For this review, take the finished solid that the model builds, in its own axes (mm). A direction names the side the tool comes from. Round coordinates to 2 decimals unless told otherwise and drop trailing zeros. Order: outer loops, then holes, each group sorted by start corner. A loop starts at its lowest first (then second) coordinate and runs counter-clockwise, first axis right, second up. Notation, with made-up numbers: M 73.5,-22.5 L 98.5,-22.5 A28 cw 98.5,14.5 Z; hole C -4.5,-20.5 d4. An arc over 180 degrees is marked long. Put each result on its own line as item: value.
from build123d import *

# Parameters (mm, degrees)
BOSS_EXTRUDE1_DEPTH = 9.95
SKETCH2_W           = 58
SKETCH2_H           = 9.95
BOSS_EXTRUDE2_DEPTH = 8.55
SKETCH3_W           = 9.8
SKETCH3_H           = 11.55
BOSS_EXTRUDE3_DEPTH = 4
BOSS_EXTRUDE4_DEPTH = 20
CHAMFER1_SIZE       = 2
CUT_EXTRUDE1_REACH  = 70.57
CHAMFER2_SIZE       = 1
BOSS_EXTRUDE5_DEPTH = 5
CHAMFER3_SIZE       = 2
SKETCH7_W           = 10
SKETCH7_H           = 20
CUT_EXTRUDE2_DEPTH  = 7
CHAMFER4_SIZE       = 2
CHAMFER5_SIZE       = 1
SKETCH8_R           = 1.25
CUT_EXTRUDE3_DEPTH  = 15
CHAMFER6_SIZE       = 1.5
CHAMFER7_SIZE       = 2


with BuildPart() as part:
    # Sketch1 → Boss-Extrude1 (new body)
    with BuildSketch(Plane(origin=(0, 0, 0), x_dir=(1, 0, 0), z_dir=(0, 1, 0))):
        with BuildLine():
            Line((-10.05, -13), (-19.52904451, -13))
            ThreePointArc((-19.52904451, -13), (-23.22122875, -23.900809511), (-29, -33.853983643))
            Line((-29, -33.853983643), (-29, -45))
            Line((-29, -45), (29, -45))
            Line((29, -45), (29, -33.853983643))
            ThreePointArc((29, -33.853983643), (23.22122875, -23.900809511), (19.52904451, -13))
            Line((19.52904451, -13), (10.05, -13))
            Line((10.05, -13), (10.05, -15.9))
            Line((10.05, -15.9), (18.25, -15.9))
            Line((18.25, -15.9), (18.25, -19.68))
            Line((18.25, -19.68), (10.05, -19.68))
            Line((10.05, -19.68), (10.05, -22.68))
            Line((10.05, -22.68), (18.360244512, -22.68))
            ThreePointArc((18.360244512, -22.68), (21.116099011, -28.699201931), (24.5, -34.389082421))
            Line((24.5, -34.389082421), (24.5, -42))
            Line((24.5, -42), (-24.5, -42))
            Line((-24.5, -42), (-24.5, -34.389082421))
            ThreePointArc((-24.5, -34.389082421), (-21.116099011, -28.699201931), (-18.360244512, -22.68))
            Line((-18.360244512, -22.68), (-10.05, -22.68))
            Line((-10.05, -22.68), (-10.05, -19.68))
            Line((-10.05, -19.68), (-18.25, -19.68))
            Line((-18.25, -19.68), (-18.25, -15.9))
            Line((-18.25, -15.9), (-10.05, -15.9))
            Line((-10.05, -15.9), (-10.05, -13))
        make_face()
    extrude(amount=BOSS_EXTRUDE1_DEPTH)

    # Sketch2 → Boss-Extrude2 (add)
    with BuildSketch(Plane.XY.offset(45)):
        with Locations((0, 4.975)):
            Rectangle(SKETCH2_W, SKETCH2_H)
    extrude(amount=BOSS_EXTRUDE2_DEPTH)

    # Sketch3 → Boss-Extrude3 (add)
    with BuildSketch(Plane(origin=(0, 9.95, 0), x_dir=(1, 0, 0), z_dir=(0, 1, 0))):
        with Locations((0, -47.775)):
            Rectangle(SKETCH3_W, SKETCH3_H)
    extrude(amount=BOSS_EXTRUDE3_DEPTH)

    # Sketch4 → Boss-Extrude4 (add)
    with BuildSketch(Plane.XY.offset(53.55)):
        Polygon((-29, 9.95), (-29, 0), (29, 0), (29, 9.95), (4.9, 9.95), (4.9, 13.95), (-4.9, 13.95), (-4.9, 9.95), align=None)
    extrude(amount=BOSS_EXTRUDE4_DEPTH)

    # Chamfer1
    chamfer1_edges = [part.edges().sort_by_distance(p)[0] for p in [
        (4.9, 11.95, 42),
        (-4.9, 11.95, 42),
    ]]
    chamfer(chamfer1_edges, length=CHAMFER1_SIZE)

    # Cut-Extrude1: up to this face of the body (flat: up to its plane)
    cut_extrude1_end = Plane(part.part.faces().sort_by_distance((14.205122256, 4.975, 22.68))[0])
    # Sketch5 → Cut-Extrude1 (cut, up to the picked face)
    with BuildSketch(Plane(origin=(0, 0, 13), x_dir=(-1, 0, 0), z_dir=(0, 0, -1)), mode=Mode.PRIVATE) as cut_extrude1_sk1:
        with BuildLine():
            ThreePointArc((-14.25, 4.975), (-13, 3.725), (-11.75, 4.975))
            Line((-11.75, 4.975), (-14.25, 4.975))
        make_face()
    cut_extrude1_tool1 = split(extrude(cut_extrude1_sk1.sketch, amount=-CUT_EXTRUDE1_REACH, mode=Mode.PRIVATE), bisect_by=cut_extrude1_end, keep=Keep.BOTH, mode=Mode.PRIVATE)
    # Sketch5 → Cut-Extrude1 (cut, up to the picked face)
    with BuildSketch(Plane(origin=(0, 0, 13), x_dir=(-1, 0, 0), z_dir=(0, 0, -1)), mode=Mode.PRIVATE) as cut_extrude1_sk2:
        with BuildLine():
            Line((-14.25, 4.975), (-11.75, 4.975))
            ThreePointArc((-11.75, 4.975), (-13, 6.225), (-14.25, 4.975))
        make_face()
    cut_extrude1_tool2 = split(extrude(cut_extrude1_sk2.sketch, amount=-CUT_EXTRUDE1_REACH, mode=Mode.PRIVATE), bisect_by=cut_extrude1_end, keep=Keep.BOTH, mode=Mode.PRIVATE)
    # Sketch5 → Cut-Extrude1 (cut, up to the picked face)
    with BuildSketch(Plane(origin=(0, 0, 13), x_dir=(-1, 0, 0), z_dir=(0, 0, -1)), mode=Mode.PRIVATE) as cut_extrude1_sk3:
        with BuildLine():
            ThreePointArc((-14.25, 4.975), (-13, 3.725), (-11.75, 4.975))
            Line((-11.75, 4.975), (-14.25, 4.975))
        make_face()
    cut_extrude1_tool3 = split(extrude(cut_extrude1_sk3.sketch, amount=-CUT_EXTRUDE1_REACH, mode=Mode.PRIVATE), bisect_by=cut_extrude1_end, keep=Keep.BOTH, mode=Mode.PRIVATE)
    # Sketch5 → Cut-Extrude1 (cut, up to the picked face)
    with BuildSketch(Plane(origin=(0, 0, 13), x_dir=(-1, 0, 0), z_dir=(0, 0, -1)), mode=Mode.PRIVATE) as cut_extrude1_sk4:
        with BuildLine():
            Line((-14.25, 4.975), (-11.75, 4.975))
            ThreePointArc((-11.75, 4.975), (-13, 6.225), (-14.25, 4.975))
        make_face()
    cut_extrude1_tool4 = split(extrude(cut_extrude1_sk4.sketch, amount=-CUT_EXTRUDE1_REACH, mode=Mode.PRIVATE), bisect_by=cut_extrude1_end, keep=Keep.BOTH, mode=Mode.PRIVATE)
    # Sketch5 → Cut-Extrude1 (cut, up to the picked face)
    with BuildSketch(Plane(origin=(0, 0, 13), x_dir=(-1, 0, 0), z_dir=(0, 0, -1)), mode=Mode.PRIVATE) as cut_extrude1_sk5:
        with BuildLine():
            ThreePointArc((14.25, 4.975), (13, 6.225), (11.75, 4.975))
            Line((11.75, 4.975), (14.25, 4.975))
        make_face()
    cut_extrude1_tool5 = split(extrude(cut_extrude1_sk5.sketch, amount=-CUT_EXTRUDE1_REACH, mode=Mode.PRIVATE), bisect_by=cut_extrude1_end, keep=Keep.BOTH, mode=Mode.PRIVATE)
    # Sketch5 → Cut-Extrude1 (cut, up to the picked face)
    with BuildSketch(Plane(origin=(0, 0, 13), x_dir=(-1, 0, 0), z_dir=(0, 0, -1)), mode=Mode.PRIVATE) as cut_extrude1_sk6:
        with BuildLine():
            Line((14.25, 4.975), (11.75, 4.975))
            ThreePointArc((11.75, 4.975), (13, 3.725), (14.25, 4.975))
        make_face()
    cut_extrude1_tool6 = split(extrude(cut_extrude1_sk6.sketch, amount=-CUT_EXTRUDE1_REACH, mode=Mode.PRIVATE), bisect_by=cut_extrude1_end, keep=Keep.BOTH, mode=Mode.PRIVATE)
    # Sketch5 → Cut-Extrude1 (cut, up to the picked face)
    with BuildSketch(Plane(origin=(0, 0, 13), x_dir=(-1, 0, 0), z_dir=(0, 0, -1)), mode=Mode.PRIVATE) as cut_extrude1_sk7:
        with BuildLine():
            ThreePointArc((14.25, 4.975), (13, 6.225), (11.75, 4.975))
            Line((11.75, 4.975), (14.25, 4.975))
        make_face()
    cut_extrude1_tool7 = split(extrude(cut_extrude1_sk7.sketch, amount=-CUT_EXTRUDE1_REACH, mode=Mode.PRIVATE), bisect_by=cut_extrude1_end, keep=Keep.BOTH, mode=Mode.PRIVATE)
    # Sketch5 → Cut-Extrude1 (cut, up to the picked face)
    with BuildSketch(Plane(origin=(0, 0, 13), x_dir=(-1, 0, 0), z_dir=(0, 0, -1)), mode=Mode.PRIVATE) as cut_extrude1_sk8:
        with BuildLine():
            Line((14.25, 4.975), (11.75, 4.975))
            ThreePointArc((11.75, 4.975), (13, 3.725), (14.25, 4.975))
        make_face()
    cut_extrude1_tool8 = split(extrude(cut_extrude1_sk8.sketch, amount=-CUT_EXTRUDE1_REACH, mode=Mode.PRIVATE), bisect_by=cut_extrude1_end, keep=Keep.BOTH, mode=Mode.PRIVATE)
    add(cut_extrude1_tool1.solids().sort_by(Axis((13, 4.444484, 13), (0, 0, 1)))[0], mode=Mode.SUBTRACT)
    add(cut_extrude1_tool2.solids().sort_by(Axis((13, 5.505516, 13), (0, 0, 1)))[0], mode=Mode.SUBTRACT)
    add(cut_extrude1_tool3.solids().sort_by(Axis((13, 4.444484, 13), (0, 0, 1)))[0], mode=Mode.SUBTRACT)
    add(cut_extrude1_tool4.solids().sort_by(Axis((13, 5.505516, 13), (0, 0, 1)))[0], mode=Mode.SUBTRACT)
    add(cut_extrude1_tool5.solids().sort_by(Axis((-13, 5.505516, 13), (0, 0, 1)))[0], mode=Mode.SUBTRACT)
    add(cut_extrude1_tool6.solids().sort_by(Axis((-13, 4.444484, 13), (0, 0, 1)))[0], mode=Mode.SUBTRACT)
    add(cut_extrude1_tool7.solids().sort_by(Axis((-13, 5.505516, 13), (0, 0, 1)))[0], mode=Mode.SUBTRACT)
    add(cut_extrude1_tool8.solids().sort_by(Axis((-13, 4.444484, 13), (0, 0, 1)))[0], mode=Mode.SUBTRACT)

    # Chamfer2
    chamfer2_edges = [part.edges().sort_by_distance(p)[0] for p in [
        (11.75, 4.975, 13),
        (-11.75, 4.975, 13),
    ]]
    chamfer(chamfer2_edges, length=CHAMFER2_SIZE)

    # Sketch6 → Boss-Extrude5 (add)
    with BuildSketch(Plane.XY.offset(73.55)):
        Polygon((29, 9.95), (29, 0), (38, 0), (38, 13.95), (4.9, 13.95), (4.9, 9.95), align=None)
        Polygon((-38, 13.95), (-38, 0), (-29, 0), (-29, 9.95), (-4.9, 9.95), (-4.9, 13.95), align=None)
    extrude(amount=-BOSS_EXTRUDE5_DEPTH)

    # Chamfer3
    chamfer3_edges = [part.edges().sort_by_distance(p)[0] for p in [
        (0, 13.95, 42),
        (3.9, 13.95, 43),
        (-3.9, 13.95, 43),
        (4.9, 13.95, 56.275),
        (33.5, 0, 68.55),
        (38, 0, 71.05),
        (38, 6.975, 68.55),
        (38, 13.95, 71.05),
        (4.9, 11.95, 68.55),
        (21.45, 13.95, 68.55),
        (-4.9, 13.95, 56.275),
        (-38, 13.95, 71.05),
        (-33.5, 0, 68.55),
        (-38, 0, 71.05),
        (-21.45, 13.95, 68.55),
        (-4.9, 11.95, 68.55),
        (-38, 6.975, 68.55),
    ]]
    chamfer(chamfer3_edges, length=CHAMFER3_SIZE)

    # Sketch7 → Cut-Extrude2 (cut)
    with BuildSketch(Plane(origin=(0, 9.95, 0), x_dir=(1, 0, 0), z_dir=(0, 1, 0))):
        with Locations((-14.9, -52)):
            Rectangle(SKETCH7_W, SKETCH7_H)
        with Locations((14.9, -52)):
            Rectangle(SKETCH7_W, SKETCH7_H)
    extrude(amount=-CUT_EXTRUDE2_DEPTH, mode=Mode.SUBTRACT)

    # Chamfer4
    chamfer4_edges = [part.edges().sort_by_distance(p)[0] for p in [
        (-9.9, 9.95, 52),
        (-9.9, 6.45, 42),
        (-9.9, 6.45, 62),
        (-19.9, 6.45, 62),
        (-19.9, 6.45, 42),
        (-19.9, 9.95, 52),
        (-14.9, 9.95, 62),
        (19.9, 9.95, 52),
        (19.9, 6.45, 42),
        (19.9, 6.45, 62),
        (9.9, 6.45, 62),
        (9.9, 6.45, 42),
        (9.9, 9.95, 52),
        (14.9, 9.95, 62),
    ]]
    chamfer(chamfer4_edges, length=CHAMFER4_SIZE)

    # Chamfer5
    chamfer5_edges = [part.edges().sort_by_distance(p)[0] for p in [
        (-24.5, 4.975, 42),
        (24.5, 4.975, 42),
    ]]
    chamfer(chamfer5_edges, length=CHAMFER5_SIZE)

    # Sketch8 → Cut-Extrude3 (cut)
    with BuildSketch(Plane.XY.offset(73.55)):
        with Locations((-25, 6.975)):
            Circle(SKETCH8_R)
        with Locations((25, 6.975)):
            Circle(SKETCH8_R)
        with Locations((0, 6.975)):
            Circle(SKETCH8_R)
    extrude(amount=-CUT_EXTRUDE3_DEPTH, mode=Mode.SUBTRACT)

    # Chamfer6
    chamfer6_edges = [part.edges().sort_by_distance(p)[0] for p in [
        (-29, 9.95, 51.201991821),
        (-14.789522255, 9.95, 13),
        (-23.22122875, 9.95, 23.900809511),
        (29, 9.95, 51.201991821),
        (23.22122875, 9.95, 23.900809511),
        (14.789522255, 9.95, 13),
    ]]
    chamfer(chamfer6_edges, length=CHAMFER6_SIZE)

    # Chamfer7
    chamfer7_edges = [part.edges().sort_by_distance(p)[0] for p in [
        (-14.9, 2.95, 42),
        (14.9, 2.95, 42),
    ]]
    chamfer(chamfer7_edges, length=CHAMFER7_SIZE)


solid = part.part
(1) Add section A-A on x = 13. State how many separate pieces and enclosed holes the cut face has, then the cut area to 3 significant figures.
A:
separate pieces: 5
enclosed holes: 0
area: 230 mm2
(2) For faces 4 (the face through (-12.08, 5.82, 14.94)), 5 (the face through (-32.55, 1.01, 69.54)), 6 (the face through (-15, 5, 62)), 7 (the face through (-28.26, 9.19, 51.44)), 8 (the face through (18.25, 5, 18)), list the 3-axis set-ups (+Z, -Z, +X, -X, +Y, -Y) from which the entire face can be reached by the end or side of a thin tool; tool diameter is ignored.
A:
face 4: -Z
face 5: -Z, -X, -Y
face 6: +Y
face 7: -Z, -X, +Y
face 8: +Y, -Y
(3) To check wall thickness, follow L1, parallel to Z at x = -16, y = 6.5; L2, parallel to X at y = 5, z = 49; L3, parallel to Y at x = -25, z = 68 (3 decimals). State the ranges of each line that lie inside material, in increasing order.
A:
L1: z = 13 to 15.9, 19.68 to 22.68, 62 to 73.55
L2: x = -29 to -19.9, -9.9 to 9.9, 19.9 to 29
L3: y = 0 to 5.725, 8.225 to 9.95
(4) Add section D-D on y = 13. Give the boundary of the cut face in (x, z).
A:
outline: M -36.95,70.55 L -36,69.6 L -6.9,69.6 L -3.85,66.55 L -3.85,44.43 L -2.47,43.05 L 2.47,43.05 L 3.85,44.43 L 3.85,66.55 L 6.9,69.6 L 36,69.6 L 36.95,70.55 L 36.95,73.55 L -36.95,73.55 Z
(5) Insertion check: pin 1 Ø2.5 at (y, z) = (3.5, 14.5) entering from +X; pin 2 Ø4 at (y, z) = (6.5, 54) entering from +X; pin 3 Ø5.5 at (x, y) = (14.5, 6.5) entering from -Z; pin 4 Ø10 at (x, z) = (-11, 38.5) entering from +Y. Each pin has a flat end and moves straight along its axis. Give the tip position at first contact, or say it passes through.
A:
pin 1: stops at x = 20.24
pin 2: stops at x = 29
pin 3: stops at z = 13
pin 4: stops at y = 9.95
(6) Add section B-B on z = 63. Give the boundary of the cut face in (x, y) (3 decimals).
A:
outline: M -29,0 L 29,0 L 29,8.45 L 27.5,9.95 L 18.9,9.95 L 17.9,8.95 L 11.9,8.95 L 10.9,9.95 L 4.9,9.95 L 4.9,11.95 L 2.9,13.95 L -2.9,13.95 L -4.9,11.95 L -4.9,9.95 L -10.9,9.95 L -11.9,8.95 L -17.9,8.95 L -18.9,9.95 L -27.5,9.95 L -29,8.45 Z; hole C -25,6.975 d2.5; hole C 0,6.975 d2.5; hole C 25,6.975 d2.5
(7) Add section C-C on x = 0. Give the boundary of the cut face in (y, z) (3 decimals).
A:
outline: M 0,42 L 11.95,42 L 13.95,44 L 13.95,73.55 L 8.225,73.55 L 8.225,58.55 L 5.725,58.55 L 5.725,73.55 L 0,73.55 Z
(8) Draft analysis for pull direction Z (two halves, no side actions). For faces 1 (the face through (28.26, 9.19, 50.96)), 2 (the face through (-37.01, 7.04, 69.56)), 3 (the face through (19.48, 9.16, 61.63)), state which applies: released by +Z, released by -Z, zero draft, split by the parting line, or undercut.
A:
face 1: zero draft
face 2: released by -Z
face 3: undercut
